CAD build for the part. Positions are in the model's coordinates, mm. A direction names the side the tool comes from. Coordinates: 2 decimals unless noted, no trailing zeros. Loops run counter-clockwise (first coordinate to the right, second up) from the corner with the lowest first, then second, coordinate; pieces in that order, holes last. Notation, with made-up numbers: (-21.75, 56.5) -> (3.25, 56.5) arc R13 ccw to (3.25, 78.5) -> close; hole circle Ø4 at (63.25, -33). An arc over 180 degrees is marked (long way). Write each question's results on one line, items separated by ' | '.
```python
from build123d import *

# Parameters (mm, degrees)
F0_W     = 108
F0_H     = 155.5
F1_DEPTH = 70
F2_R     = 6.5
F3_DEPTH = 70.001
F4_W     = 50
F4_H     = 25
F5_DEPTH = 70.001
F6_R     = 10
F7_DEPTH = 20
F8_W     = 20
F8_H     = 42.75
F8_H_2   = 20
F8_W_2   = 44
F9_DEPTH = 5


with BuildPart() as f1:
    # F0 (on Right) → F1 (new body)
    with BuildSketch(Plane.YZ):
        Rectangle(F0_W, F0_H)
    extrude(amount=-F1_DEPTH)

    # F2 (on face) → F3 (cut, through all)
    with BuildSketch(Plane(origin=(-70, 0, 0), x_dir=(0, -1, 0), z_dir=(-1, 0, 0))):
        with Locations((-42, 47)):
            Circle(F2_R)
        with Locations((42, 47)):
            Circle(F2_R)
        with Locations((-42, -47)):
            Circle(F2_R)
        with Locations((42, -47)):
            Circle(F2_R)
    extrude(amount=-F3_DEPTH, mode=Mode.SUBTRACT)

    # F4 (on face) → F5 (cut, through all)
    with BuildSketch(Plane(origin=(-70, 0, 0), x_dir=(0, -1, 0), z_dir=(-1, 0, 0))):
        with Locations((0, 65.25)):
            Rectangle(F4_W, F4_H)
        with Locations((0, -65.25)):
            Rectangle(F4_W, F4_H)
    extrude(amount=-F5_DEPTH, mode=Mode.SUBTRACT)

    # F6 (on face) → F7 (cut)
    with BuildSketch(Plane(origin=(-70, 0, 0), x_dir=(0, -1, 0), z_dir=(-1, 0, 0))):
        with Locations((-42, 47)):
            Circle(F6_R)
        with Locations((-42, -47)):
            Circle(F6_R)
        with Locations((42, 47)):
            Circle(F6_R)
        with Locations((42, -47)):
            Circle(F6_R)
    extrude(amount=-F7_DEPTH, mode=Mode.SUBTRACT)

    # F8 (on face) → F9 (cut)
    with BuildSketch(Plane.YZ):
        with Locations((0, 31.375)):
            Rectangle(F8_W, F8_H)
        Rectangle(F8_W, F8_H_2)
        with Locations((-32, 0)):
            Rectangle(F8_W_2, F8_H_2)
        with Locations((32, 0)):
            Rectangle(F8_W_2, F8_H_2)
        with Locations((0, -31.375)):
            Rectangle(F8_W, F8_H)
    extrude(amount=-F9_DEPTH, mode=Mode.SUBTRACT)


solid = f1.part
```
Q1. Cut at C-C on x = -44.5. Write the cut outline in (y, z).
Results are:
outline: (-54, -77.75) -> (-25, -77.75) -> (-25, -52.75) -> (25, -52.75) -> (25, -77.75) -> (54, -77.75) -> (54, 77.75) -> (25, 77.75) -> (25, 52.75) -> (-25, 52.75) -> (-25, 77.75) -> (-54, 77.75) -> close; hole circle Ø13 at (-42, -47); hole circle Ø13 at (-42, 47); hole circle Ø13 at (42, -47); hole circle Ø13 at (42, 47)
Q2. Cut at D-D on y = -14.5. Write the cut outline in (x, z).
Results are:
outline: (-70, -52.75) -> (0, -52.75) -> (0, -10) -> (-5, -10) -> (-5, 10) -> (0, 10) -> (0, 52.75) -> (-70, 52.75) -> close
Q3. Wall check: L1, parallel to Z at x = -57.5, y = -42; L2, parallel to Z at x = -40, y = -42; L3, parallel to Y at x = -48, z = 71. Give the ranges that are in metal, low to high. Write a range as from..to.
Results are:
L1: -77.75..-57, -37..37, 57..77.75 | L2: -77.75..-53.5, -40.5..40.5, 53.5..77.75 | L3: -54..-25, 25..54
Q4. Cut at B-B on y = -42. Write the cut outline in (x, z).
Results are:
outline: (-70, -77.75) -> (0, -77.75) -> (0, -53.5) -> (-50, -53.5) -> (-50, -57) -> (-70, -57) -> close; (-70, -37) -> (-50, -37) -> (-50, -40.5) -> (0, -40.5) -> (0, -10) -> (-5, -10) -> (-5, 10) -> (0, 10) -> (0, 40.5) -> (-50, 40.5) -> (-50, 37) -> (-70, 37) -> close; (-70, 57) -> (-50, 57) -> (-50, 53.5) -> (0, 53.5) -> (0, 77.75) -> (-70, 77.75) -> close
Q5. Which spindle directions (+Z, -Z, +X, -X, +Y, -Y) get a long thin tool onto all of the face, cutting with end or side? Do faces 1 (the flat face through (-2, 32, 10)), 2 (the cylindrical face through (-60.14, -39.83, 37.24)), 3 (the flat face through (-2, 10, 31)), 4 (the flat face through (-35, 39, 77.75)), 5 (the flat face through (-35, 25, -65)). Say none if no direction does.
Results are:
face 1: +X, +Y, -Y | face 2: -X | face 3: +Z, -Z, +X | face 4: +Z, +X, -X, +Y, -Y | face 5: -Z, +X, -X
Q6. Drop flat-ended pins along their axis: pin 1 (4 mm diameter, centred on x = -11, y = -7, fed in from -Z); pin 2 (8 mm diameter, centred on x = -46.5, y = -4, fed in from +Z). Give the stop position or say it passes through.
Results are:
pin 1: z = -52.75 | pin 2: z = 52.75
Q7. Cut at A-A on z = -47. Write the cut outline in (x, y).
Results are:
outline: (-70, -54) -> (0, -54) -> (0, -48.5) -> (-50, -48.5) -> (-50, -52) -> (-70, -52) -> close; (-70, -32) -> (-50, -32) -> (-50, -35.5) -> (0, -35.5) -> (0, -10) -> (-5, -10) -> (-5, 10) -> (0, 10) -> (0, 35.5) -> (-50, 35.5) -> (-50, 32) -> (-70, 32) -> close; (-70, 52) -> (-50, 52) -> (-50, 48.5) -> (0, 48.5) -> (0, 54) -> (-70, 54) -> close
Q8. Pull direction Y, two halves, no side cores. Call faces 6 (the cylindrical face through (-25.35, -36.842, -50.955)), 7 (the flat face through (-35, 54, -1)), 8 (the cylindrical face through (-60.14, -39.83, -56.76)), 9 (the flat face through (0, 32, -43)): +Y half, -Y half, draft (parallel to the pull), parting line (faces both ways), or undercut.
Results are:
face 6: undercut | face 7: +Y half | face 8: undercut | face 9: draft
